Geometry: final body of the model. Coordinates: model frame, mm. A direction names the side the tool comes from. Coordinates: 2 decimals unless noted, no trailing zeros. Write each loop counter-clockwise with the first axis right and the second up, starting at its lowest first coordinate (ties: lowest second). Pieces come first, ordered by that corner, then holes. Notation, with made-up numbers: (6, 31.25) -> (60, 31.25) arc R4 ccw to (60, 36.25) -> close; hole circle Ø2 at (0, 62). An arc over 180 degrees is marked (long way). One line per item, written item: value. Start each with the question number.
from build123d import *

# Parameters (mm, degrees)
F0_W      = 40
F0_H      = 80
F1_DEPTH  = 20.1
F2_W      = 40
F2_H      = 40
F3_DEPTH  = 10
F4_R      = 10
F5_DEPTH  = 10.1
F7_R      = 19.99999
F8_R      = 10
F9_DEPTH  = 80
F10_W     = 20.2
F10_H     = 40
F11_DEPTH = 40
F12_R     = 19.99999


# Not quite as in the source:
# - a fillet or chamfer is up to 0.001 mm smaller than in the source, because OpenCascade refuses the exact size


with BuildPart() as f1:
    # F0 (on Right) → F1 (new body)
    with BuildSketch(Plane.YZ):
        Rectangle(F0_W, F0_H)
    extrude(amount=F1_DEPTH)

    # F2 (on face) → F3 (join)
    with BuildSketch(Plane.YZ.offset(20.1)):
        with Locations((0, 60)):
            Rectangle(F2_W, F2_H)
    extrude(amount=-F3_DEPTH)

    # F4 (on face) → F5 (cut)
    with BuildSketch(Plane.YZ.offset(20.1)):
        with Locations((0, 60)):
            Circle(F4_R)
    extrude(amount=-F5_DEPTH, mode=Mode.SUBTRACT)

    # F6: F1 across face


with BuildPart() as f1_1:
    add(f1.part)
    add(f1.part.mirror(Plane(origin=(0, 0, 0), x_dir=(0, 1, 0), z_dir=(-1, 0, 0))))

    # F7 (radius 20 in the source; OpenCascade refuses exactly that, so slightly less here)
    f7_edges = [f1_1.edges().sort_by_distance(p)[0] for p in [
        (15.1, 20, 80),
        (15.1, -20, 80),
        (-15.1, 20, 80),
        (-15.1, -20, 80),
    ]]
    fillet(f7_edges, radius=F7_R)

    # F8 (on face) → F9 (cut)
    with BuildSketch(Plane(origin=(-20.1, 0, 0), x_dir=(0, -1, 0), z_dir=(-1, 0, 0))):
        with Locations((0, -20)):
            Circle(F8_R)
    extrude(amount=-F9_DEPTH, mode=Mode.SUBTRACT)

    # F10 (on face) → F11 (cut, through all)
    with BuildSketch(Plane(origin=(0, 20, 0), x_dir=(-1, 0, 0), z_dir=(0, 1, 0))):
        with Locations((0, -20)):
            Rectangle(F10_W, F10_H)
    extrude(amount=-F11_DEPTH, mode=Mode.SUBTRACT)

    # F12 (radius 20 in the source; OpenCascade refuses exactly that, so slightly less here)
    f12_edges = [f1_1.edges().sort_by_distance(p)[0] for p in [
        (-15.1, 20, -40),
        (-15.1, -20, -40),
        (15.1, 20, -40),
        (15.1, -20, -40),
    ]]
    fillet(f12_edges, radius=F12_R)


solid = f1_1.part
Q1. Cut plane B-B on z = -14. Output: boundary loops of the cut face in (x, y).
Q2. Cut plane D-D on z = 72.5. Output: boundary loops of the cut face in (x, y), and give its area (4 significant figures).
Q3. Cut plane C-C on y = -5. Output: boundary loops of the cut face in (x, z).
Q4. Draft query along X for faces 1 (the cylindrical face through (-15.03, -14.297, 73.986)), 2 (the flat face through (10.1, 0, -7)), 3 (the flat face through (10.1, 0, 47)), 4 (the flat face through (20.1, 0, 21)). Return one class per face: pulls with the +X half, pulls with the -X half, needs draft (parallel to the pull), parting line crosses it, or undercut.
Q5. Line query: L1, parallel to Z at x = -15.25, y = 0; L2, parallel to X at y = -17.5, z = 51; L3, parallel to Z at x = -18, y = -6. Output: solid intervals per line, ascending. Write a range as from..to.
Q6. Cut plane A-A on x = 12. Count the separate pieces of the cut face and the enclosed holes in it, and give its area (3 significant figures).
Q7. First-contact query: P1, Ø3, axis at x = 10.5, y = -12, coming from the -Z side; P2, Ø12, axis at y = 2, z = -21.5, coming from the -X side; P3, Ø16, axis at x = 0.5, y = -10, coming from the -Z side; P4, Ø6, axis at x = -4.5, y = -10, coming from the +Z side. Flat tips, straight axial feed; report the tip coordinate or a pass-through.
Q8. Access query for faces 5 (the flat face through (0, 0, 40)), 6 (the flat face through (0, 0, 0)), 7 (the cylindrical face through (15.17, -14.297, -33.986)). Directions: +Z, -Z, +X, -X, +Y, -Y. A direction counts if a zero-diameter tool reaches every point of the face in a straight line with its end or side. Return the directions, or none.
Solution:
1. outline: (-20.1, -20) -> (-10.1, -20) -> (-10.1, -8) -> (-20.1, -8) -> close; (-20.1, 8) -> (-10.1, 8) -> (-10.1, 20) -> (-20.1, 20) -> close; (10.1, -20) -> (20.1, -20) -> (20.1, -8) -> (10.1, -8) -> close; (10.1, 8) -> (20.1, 8) -> (20.1, 20) -> (10.1, 20) -> close
2. outline: (-20.1, -15.61) -> (-10.1, -15.61) -> (-10.1, 15.61) -> (-20.1, 15.61) -> close; (10.1, -15.61) -> (20.1, -15.61) -> (20.1, 15.61) -> (10.1, 15.61) -> close
2. area: 624.5 mm²
3. outline: (-20.1, -39.36) -> (-10.1, -39.36) -> (-10.1, -28.66) -> (-20.1, -28.66) -> close; (-20.1, -11.34) -> (-10.1, -11.34) -> (-10.1, 0) -> (10.1, 0) -> (10.1, -11.34) -> (20.1, -11.34) -> (20.1, 51.34) -> (10.1, 51.34) -> (10.1, 40) -> (-10.1, 40) -> (-10.1, 51.34) -> (-20.1, 51.34) -> close; (-20.1, 68.66) -> (-10.1, 68.66) -> (-10.1, 79.36) -> (-20.1, 79.36) -> close; (10.1, -39.36) -> (20.1, -39.36) -> (20.1, -28.66) -> (10.1, -28.66) -> close; (10.1, 68.66) -> (20.1, 68.66) -> (20.1, 79.36) -> (10.1, 79.36) -> close
4. face 1: needs draft
4. face 2: undercut
4. face 3: undercut
4. face 4: pulls with the +X half
5. L1: -40..-30, -10..50, 70..80
5. L2: -20.1..-10.1, 10.1..20.1
5. L3: -39.08..-28, -12..52, 68..79.08
6. separate pieces: 1
6. enclosed holes: 2
6. area: 3,830 mm²
7. P1: z = -37.02
7. P2: through
7. P3: z = 0
7. P4: z = 40
8. face 5: +Z, +Y, -Y
8. face 6: -Z, +Y, -Y
8. face 7: -Z, +X, -X, -Y
